Verification items for the finished model (mm, model axes). A direction names the side the tool comes from. Round coordinates to 2 decimals unless told otherwise and drop trailing zeros. Write each loop counter-clockwise with the first axis right and the second up, starting at its lowest first coordinate (ties: lowest second). Pieces come first, ordered by that corner, then holes. Notation, with made-up numbers: M 71,81 L 92,81 A12 ccw 92,100 Z; hole C 29,44.5 d1. An arc over 180 degrees is marked long. One line per question, with ' | ' between items. Start each with the question number.
Q1. Cross-section at B-B (y = 14). Record the boundary of the cut face in (x, z) (3 decimals).
Q2. Tool access check on faces 1 (the face through (49, 3, 3)), 2 (the face through (1, -34.5, 3)), 3 (the face through (-1, -31, 4.84)). Record the directions out of +Z, -Z, +X, -X, +Y, -Y that give a thin tool (end or side, any length) a straight path to the whole face; none if there is none.
Q3. Release check for a two-part mould opening along X. For faces 4 (the face through (-47.7, -34, -1.7)), 5 (the face through (-49, 3, 3)), 6 (the face through (-1, -35.575, 1)) record: released by +X, released by -X, zero draft, split by the parting line, or undercut.
Q4. Cross-section at D-D (y = -30). Record the boundary of the cut face in (x, z) (3 decimals), then the cut area to 3 significant figures.
Q5. Cross-section at C-C (x = 8). Record the boundary of the cut face in (y, z) (3 decimals), then the cut area to 3 significant figures.
Q6. Cross-section at A-A (x = -43.5). Record the boundary of the cut face in (y, z) (3 decimals), then the cut area to 3 significant figures.
Q7. Thickness scan on line 1 along Z through (x, y) = (16.5, -11); line 2 along Y through (x, z) = (36, 4.75) (3 decimals); line 3 along Y through (x, z) = (26.5, -2.25). Record the ranges inside material, lowest first. Write a range as from..to.
Q8. Gauge pin test, flat ends, axial feed: pin 1 (0.9 mm diameter, centred on y = 5.5, z = 4, fed in from +X); pin 2 (12 mm diameter, centred on x = 16.5, y = 20, fed in from -Z); pin 3 (5 mm diameter, centred on x = 27, y = -21, fed in from +Z). Record the tip position at first contact, or that the pin passes through.
from build123d import *

# Parameters (mm, degrees)
ESQUISSE2_W                  = 100.15
ESQUISSE2_H                  = 71.15
BOSS_EXTRU_1_DEPTH           = 5
ESQUISSE3_W                  = 98
ESQUISSE3_H                  = 69
ENL_V_MAT_EXTRU_1_DEPTH      = 0.08
ESQUISSE4_W                  = 98
ESQUISSE4_H                  = 6.140882506
ENL_V_MAT_EXTRU_2_DEPTH      = 0.08
ESQUISSE5_W                  = 80.249689796
ESQUISSE5_H                  = 1.075
ENL_V_MAT_EXTRU_3_DEPTH      = 3
CONG_1_R                     = 0.5
CONG_2_R                     = 0.5
ESQUISSE7_W                  = 1.075
ESQUISSE7_H                  = 12.243191877
ENL_V_MAT_EXTRU_4_DEPTH      = 3
ESQUISSE8_R                  = 1
BOSS_EXTRU_3_DEPTH           = 4
BOSS_EXTRU_3_DRAFT           = 4
BOSS_EXTRU_3_PROFILE_2_DEPTH = 4
BOSS_EXTRU_3_PROFILE_2_DRAFT = 4
BOSS_EXTRU_3_PROFILE_3_DEPTH = 4
BOSS_EXTRU_3_PROFILE_3_DRAFT = 4
BOSS_EXTRU_3_PROFILE_4_DEPTH = 4
BOSS_EXTRU_3_PROFILE_4_DRAFT = 4
CONG_3_R                     = 0.5
CONG_4_R                     = 0.5
CONG_5_R                     = 0.5
CONG_6_R                     = 0.5
ESQUISSE9_R                  = 0.15
BOSS_EXTRU_5_DEPTH           = 4


with BuildPart() as part:
    # Esquisse2 → Boss.-Extru.1 (new body)
    with BuildSketch(Plane.XY):
        Rectangle(ESQUISSE2_W, ESQUISSE2_H)
    extrude(amount=BOSS_EXTRU_1_DEPTH)

    # Esquisse3 → Enlèv. mat.-Extru.1 (cut)
    with BuildSketch(Plane.XY.offset(5)):
        Rectangle(ESQUISSE3_W, ESQUISSE3_H)
    extrude(amount=-ENL_V_MAT_EXTRU_1_DEPTH, mode=Mode.SUBTRACT)

    # Esquisse4 → Enlèv. mat.-Extru.2 (cut)
    with BuildSketch(Plane.XY.offset(4.92)):
        with Locations((0, -31.429558747)):
            Rectangle(ESQUISSE4_W, ESQUISSE4_H)
    extrude(amount=-ENL_V_MAT_EXTRU_2_DEPTH, mode=Mode.SUBTRACT)

    # Esquisse5 → Enlèv. mat.-Extru.3 (cut)
    with BuildSketch(Plane.XY.offset(5)):
        with Locations((-0.000155102, -35.0375)):
            Rectangle(ESQUISSE5_W, ESQUISSE5_H)
    extrude(amount=-ENL_V_MAT_EXTRU_3_DEPTH, mode=Mode.SUBTRACT)

    # Congé1
    # the kernel refuses this fillet: 0.5 mm, written as the material it takes off along each edge
    with BuildSketch(Plane(origin=(-40.125, -36.825, 5), x_dir=(-1, 0, 0), z_dir=(0, 1, 0))) as cong_1_piece_1:
        with BuildLine():
            CenterArc((CONG_1_R, -CONG_1_R), CONG_1_R, 90, 90)
            Line((0, -CONG_1_R), (0, 0))
            Line((0, 0), (CONG_1_R, 0))
        make_face()
    extrude(amount=2.325, mode=Mode.SUBTRACT)

    # Congé2
    # the kernel refuses this fillet: 0.5 mm, written as the material it takes off along each edge
    with BuildSketch(Plane(origin=(40.124689796, -34.5, 5), x_dir=(0, 0, -1), z_dir=(0, -1, 0))) as cong_2_piece_1:
        with BuildLine():
            CenterArc((CONG_2_R, CONG_2_R), CONG_2_R, 180, 90)
            Line((0, CONG_2_R), (0, 0))
            Line((0, 0), (CONG_2_R, 0))
        make_face()
    extrude(amount=2.325, mode=Mode.SUBTRACT)

    # Esquisse7 → Enlèv. mat.-Extru.4 (cut)
    with BuildSketch(Plane.XY.offset(5)):
        with Locations((-49.5375, 3.433132672)):
            Rectangle(ESQUISSE7_W, ESQUISSE7_H)
        with Locations((49.5375, 3.433132672)):
            Rectangle(ESQUISSE7_W, ESQUISSE7_H)
    extrude(amount=-ENL_V_MAT_EXTRU_4_DEPTH, mode=Mode.SUBTRACT)


with BuildPart() as boss_extru_3_tool:
    # Esquisse8 → Boss.-Extru.3 (with draft: the straight prism first)
    with BuildSketch(Plane(origin=(0, 0, 0), x_dir=(-1, 0, 0), z_dir=(0, 0, -1))):
        with Locations((-48.577420287, -34.074984175)):
            Circle(ESQUISSE8_R)
    extrude(amount=BOSS_EXTRU_3_DEPTH)
    # Boss.-Extru.3: the draft: its side faces are tilted about the plane it starts from
    boss_extru_3_sides = [boss_extru_3_tool.faces().sort_by_distance(p)[0] for p in [
        (49.577420287, -34.074984175, -2),
    ]]
    draft(boss_extru_3_sides, Plane(origin=(0, 0, 0), x_dir=(-1, 0, 0), z_dir=(0, 0, -1)), BOSS_EXTRU_3_DRAFT)


with BuildPart() as part_1:
    add(part.part)

    # Boss.-Extru.3: add boss_extru_3_tool
    add(boss_extru_3_tool.part)


with BuildPart() as boss_extru_3_profile_2_tool:
    # Esquisse8 → Boss.-Extru.3 profile 2 (with draft: the straight prism first)
    with BuildSketch(Plane(origin=(0, 0, 0), x_dir=(-1, 0, 0), z_dir=(0, 0, -1))):
        with Locations((-48.577420287, 34.07588992)):
            Circle(ESQUISSE8_R)
    extrude(amount=BOSS_EXTRU_3_PROFILE_2_DEPTH)
    # Boss.-Extru.3 profile 2: the draft: its side faces are tilted about the plane it starts from
    boss_extru_3_profile_2_sides = [boss_extru_3_profile_2_tool.faces().sort_by_distance(p)[0] for p in [
        (49.577420287, 34.07588992, -2),
    ]]
    draft(boss_extru_3_profile_2_sides, Plane(origin=(0, 0, 0), x_dir=(-1, 0, 0), z_dir=(0, 0, -1)), BOSS_EXTRU_3_PROFILE_2_DRAFT)


with BuildPart() as part_2:
    add(part_1.part)

    # Boss.-Extru.3 profile 2: add boss_extru_3_profile_2_tool
    add(boss_extru_3_profile_2_tool.part)


with BuildPart() as boss_extru_3_profile_3_tool:
    # Esquisse8 → Boss.-Extru.3 profile 3 (with draft: the straight prism first)
    with BuildSketch(Plane(origin=(0, 0, 0), x_dir=(-1, 0, 0), z_dir=(0, 0, -1))):
        with Locations((48.578218454, 34.07588992)):
            Circle(ESQUISSE8_R)
    extrude(amount=BOSS_EXTRU_3_PROFILE_3_DEPTH)
    # Boss.-Extru.3 profile 3: the draft: its side faces are tilted about the plane it starts from
    boss_extru_3_profile_3_sides = [boss_extru_3_profile_3_tool.faces().sort_by_distance(p)[0] for p in [
        (-47.578218454, 34.07588992, -2),
    ]]
    draft(boss_extru_3_profile_3_sides, Plane(origin=(0, 0, 0), x_dir=(-1, 0, 0), z_dir=(0, 0, -1)), BOSS_EXTRU_3_PROFILE_3_DRAFT)


with BuildPart() as part_3:
    add(part_2.part)

    # Boss.-Extru.3 profile 3: add boss_extru_3_profile_3_tool
    add(boss_extru_3_profile_3_tool.part)


with BuildPart() as boss_extru_3_profile_4_tool:
    # Esquisse8 → Boss.-Extru.3 profile 4 (with draft: the straight prism first)
    with BuildSketch(Plane(origin=(0, 0, 0), x_dir=(-1, 0, 0), z_dir=(0, 0, -1))):
        with Locations((48.578218454, -34.074984175)):
            Circle(ESQUISSE8_R)
    extrude(amount=BOSS_EXTRU_3_PROFILE_4_DEPTH)
    # Boss.-Extru.3 profile 4: the draft: its side faces are tilted about the plane it starts from
    boss_extru_3_profile_4_sides = [boss_extru_3_profile_4_tool.faces().sort_by_distance(p)[0] for p in [
        (-47.578218454, -34.074984175, -2),
    ]]
    draft(boss_extru_3_profile_4_sides, Plane(origin=(0, 0, 0), x_dir=(-1, 0, 0), z_dir=(0, 0, -1)), BOSS_EXTRU_3_PROFILE_4_DRAFT)


with BuildPart() as part_4:
    add(part_3.part)

    # Boss.-Extru.3 profile 4: add boss_extru_3_profile_4_tool
    add(boss_extru_3_profile_4_tool.part)

    # Congé3
    cong_3_edges = [part_4.edges().sort_by_distance(p)[0] for p in [
        (49.297713039, 34.07588992, -4),
    ]]
    fillet(cong_3_edges, radius=CONG_3_R)

    # Congé4
    cong_4_edges = [part_4.edges().sort_by_distance(p)[0] for p in [
        (-47.857925701, 34.07588992, -4),
    ]]
    fillet(cong_4_edges, radius=CONG_4_R)

    # Congé5
    cong_5_edges = [part_4.edges().sort_by_distance(p)[0] for p in [
        (-47.857925701, -34.074984175, -4),
    ]]
    fillet(cong_5_edges, radius=CONG_5_R)

    # Congé6
    cong_6_edges = [part_4.edges().sort_by_distance(p)[0] for p in [
        (49.297713039, -34.074984175, -4),
    ]]
    fillet(cong_6_edges, radius=CONG_6_R)

    # Esquisse9 → Boss.-Extru.5 (add)
    with BuildSketch(Plane(origin=(0, 0, 0), x_dir=(-1, 0, 0), z_dir=(0, 0, -1))):
        with Locations((26.5, -34.476200763)):
            Circle(ESQUISSE9_R)
        with Locations((-26.5, -34.476200763)):
            Circle(ESQUISSE9_R)
    extrude(amount=BOSS_EXTRU_5_DEPTH)


solid = part_4.part
Determined:
1) outline: M -50.075,0 L 50.075,0 L 50.075,5 L 49,5 L 49,4.92 L -49,4.92 L -49,5 L -50.075,5 Z
2) face 1: +Z, +X | face 2: +Z, -Y | face 3: +Z
3) face 4: undercut | face 5: released by -X | face 6: zero draft
4) outline: M -50.075,0 L 50.075,0 L 50.075,5 L 49,5 L 49,4.84 L -49,4.84 L -49,5 L -50.075,5 Z | area: 485 mm²
5) outline: M -35.575,0 L 35.575,0 L 35.575,5 L 34.5,5 L 34.5,4.92 L -28.359,4.92 L -28.359,4.84 L -34.5,4.84 L -34.5,2 L -35.575,2 Z | area: 347 mm²
6) outline: M -35.575,0 L 35.575,0 L 35.575,5 L 34.5,5 L 34.5,4.92 L -28.359,4.92 L -28.359,4.84 L -34.5,4.84 L -34.5,5 L -35.575,5 Z | area: 350 mm²
7) line 1: z = 0..4.92 | line 2: y = -34.5..35.575 | line 3: y = -34.63..-34.33
8) pin 1: stops at x = 49 | pin 2: stops at z = 0 | pin 3: stops at z = 4.92
